```python
from build123d import *

# Parameters (mm, degrees)
BOSS_EXTRUDE2_DEPTH   = 30
F_3_0MM_DOWEL_HOLE1_D = 24


with BuildPart() as part:
    # Sketch1 → Boss-Extrude2 (new body)
    with BuildSketch(Plane.XY):
        with BuildLine():
            Line((0, 25), (800, 25))
            ThreePointArc((800, 25), (825, 0), (800, -25))
            Line((800, -25), (0, -25))
            ThreePointArc((0, -25), (-25, 0), (0, 25))
        make_face()
    extrude(amount=BOSS_EXTRUDE2_DEPTH)

    # Ø3.0mm Dowel Hole1 (through all)
    with Locations(Plane.XY.offset(30)):
        with Locations((0, 0), (800, 0), (400, 0)):
            Hole(F_3_0MM_DOWEL_HOLE1_D / 2)


solid = part.part
```
Build history of the part. All positions in model axes, mm. Round coordinates to 2 decimals unless told otherwise and drop trailing zeros. Write each loop counter-clockwise with the first axis right and the second up, starting at its lowest first coordinate (ties: lowest second). Pieces come first, ordered by that corner, then holes.
1) Band-saw the part on B-B, the plane y = 0. List the corners of the cut face in (x, z), and give its area (3 significant figures).
2) Pin check, flat tips, straight feed: pin 1 (1.5 mm diameter, centred on y = 3, z = 6, fed in from +X); pin 2 (10 mm diameter, centred on y = -0.5, z = 3.5, fed in from +X); pin 3 (8 mm diameter, centred on y = 16.5, z = 8.5, fed in from +X). Stop position of each tip, or through.
3) Band-saw the part on C-C, the plane z = 17.25. List the corners of the cut face in (x, y).
4) Drill centre lines: probe 1 along X at (y, z) = (1, 5); probe 2 along Y at (x, z) = (0, 20); probe 3 along X at (y, z) = (-4, 9.5). Where is each one in solid material? Low to high.
5) Mould opens along X. For faces 1 (the cylindrical face through (411.99, 0.53, 14.79)), 2 (the flat face through (394, 25, 15)), 3 (the cylindrical face through (824.994, 0.55, 14.79)), 4 (the cylindrical face through (-24.994, -0.55, 14.79)) say: +X half, -X half, draft (parallel to the pull), parting line (faces both ways), or undercut.
6) Band-saw the part on A-A, the plane x = 400. List the corners of the cut face in (y, z).
Ans:
1. outline: (-25, 0) - (-12, 0) - (-12, 30) - (-25, 30) - close; (12, 0) - (388, 0) - (388, 30) - (12, 30) - close; (412, 0) - (788, 0) - (788, 30) - (412, 30) - close; (812, 0) - (825, 0) - (825, 30) - (812, 30) - close
1. area: 23,300 mm2
2. pin 1: stops at x = 824.9
2. pin 2: stops at x = 825
2. pin 3: stops at x = 821.65
3. outline: (0, -25) - (800, -25) arc R25 ccw to (800, 25) - (0, 25) arc R25 ccw to start; hole circle Ø24 at (0, 0); hole circle Ø24 at (400, 0); hole circle Ø24 at (800, 0)
4. probe 1: x = -24.98 to -11.96, 11.96 to 388.04, 411.96 to 788.04, 811.96 to 824.98
4. probe 2: y = -25 to -12, 12 to 25
4. probe 3: x = -24.68 to -11.31, 11.31 to 388.69, 411.31 to 788.69, 811.31 to 824.68
5. face 1: undercut
5. face 2: draft
5. face 3: +X half
5. face 4: -X half
6. outline: (-25, 0) - (-12, 0) - (-12, 30) - (-25, 30) - close; (12, 0) - (25, 0) - (25, 30) - (12, 30) - close
